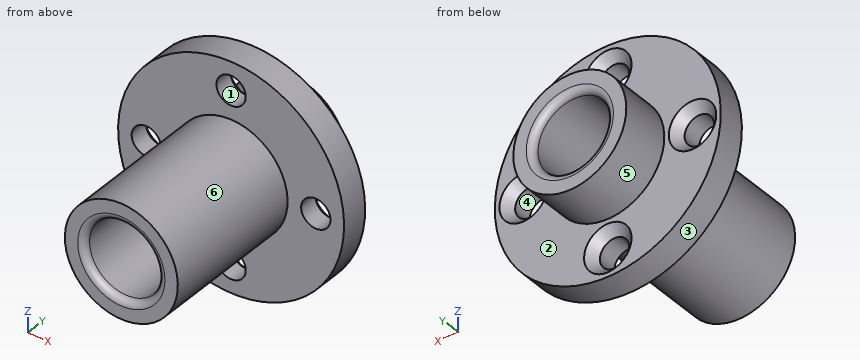
```python
from build123d import *

# Parameters (mm, degrees)
SKETCH2_R                    = 1.65
CUT_EXTRUDE1_DEPTH           = 27.647311778
CHAMFER1_SIZE                = 1.016
CIRPATTERN1_COUNT            = 4
CHAMFER1_OF_CIRPATTERN1_SIZE = 1.016
FILLET1_R                    = 0.762


with BuildPart() as part:
    # Sketch1 → Revolve1 (revolve)
    with BuildSketch(Plane.XY, mode=Mode.PRIVATE) as revolve1_sk:
        Polygon((4.1402, 12.7), (4.1402, -12.7), (6.35, -12.7), (6.35, 3.81), (12.7, 3.81), (12.7, 6.985), (6.35, 6.985), (6.35, 12.7), align=None)
    revolve(revolve1_sk.sketch.rotate(Axis((0, 0, 0), (0, -1, 0)), 90), axis=Axis((0, 0, 0), (0, -1, 0)))

    # Sketch2 → Cut-Extrude1 (cut, through all)
    with BuildSketch(Plane(origin=(0, 6.985, 0), x_dir=(1, 0, 0), z_dir=(0, 1, 0))):
        with Locations(Location((0, 9.525, 0), (0, 0, 270))):
            Circle(SKETCH2_R)
    cut_extrude1 = extrude(amount=-CUT_EXTRUDE1_DEPTH, mode=Mode.SUBTRACT)

    # Chamfer1
    chamfer1_edges = [part.edges().sort_by_distance(p)[0] for p in [
        (0, 6.985, -11.175),
    ]]
    chamfer(chamfer1_edges, length=CHAMFER1_SIZE)

    # CirPattern1: Cut-Extrude1 ×4 about axis
    cirpattern1_axis = Axis((0, 0, 0), (0, 1, 0))
    for i in range(1, CIRPATTERN1_COUNT):
        add(cut_extrude1.rotate(cirpattern1_axis, i * 360 / CIRPATTERN1_COUNT), mode=Mode.SUBTRACT)

    # Chamfer1 of CirPattern1
    chamfer1_of_cirpattern1_edges = [part.edges().sort_by_distance(p)[0] for p in [
        (-11.175, 6.985, 0),
        (0, 6.985, 11.175),
        (11.175, 6.985, 0),
    ]]
    chamfer(chamfer1_of_cirpattern1_edges, length=CHAMFER1_OF_CIRPATTERN1_SIZE)

    # Fillet1
    fillet1_edges = [part.edges().sort_by_distance(p)[0] for p in [
        (0, 12.7, -4.1402),
        (0, -12.7, -4.1402),
    ]]
    fillet(fillet1_edges, radius=FILLET1_R)


solid = part.part
```
Model file for the job. Use its own axes, mm. Face numbers are marked on the shaded views. A direction names the side the tool comes from. Round coordinates to 2 decimals unless told otherwise and drop trailing zeros. Write each loop counter-clockwise with the first axis right and the second up, starting at its lowest first coordinate (ties: lowest second). Pieces come first, ordered by that corner, then holes. Notation, with made-up numbers: M -13,-37 L 34,-37 A36 ccw 34,2 Z; hole C 21.5,79.25 d6. An arc over 180 degrees is marked long. Put each result on its own line as item: value.
Item 1: Probe L1, parallel to X at y = 3.75, z = 0; L2, parallel to Y at x = -6.5, z = -9.25 (3 decimals); L3, parallel to Z at x = -1.25, y = 2. List the from-to ranges inside material, lowest first. Write a range as from..to.
Responses:
L1: -6.35..-4.14, 4.14..6.35
L2: 3.81..6.985
L3: -6.23..-3.95, 3.95..6.23
Item 2: Cut at D-D (y = 2.5). List the corners of the cut face in (x, z), and give its area (3 significant figures).
Responses:
outline: C 0,0 d12.7; hole C 0,0 d8.28
area: 72.8 mm²
Item 3: Tool access for the marked faces 4, 5 and 6: list every direction of +Z, -Z, +X, -X, +Y, -Y with a clear straight run to the whole face (end or side of a thin tool).
Responses:
face 4: +Y, -Y
face 5: +Y
face 6: -Y
Item 4: Cut at C-C (x = 5.5). List the corners of the cut face in (y, z) (3 decimals), and give its area (3 significant figures).
Responses:
outline: M -12.7,-3.174 L 3.81,-3.174 L 3.81,-11.447 L 6.985,-11.447 L 6.985,-3.174 L 12.7,-3.174 L 12.7,3.174 L 6.985,3.174 L 6.985,11.447 L 3.81,11.447 L 3.81,3.174 L -12.7,3.174 Z
area: 214 mm²
Item 5: Cut at A-A (z = 0). State how many separate pieces and enclosed holes the cut face has, and give its area (3 significant figures).
Responses:
separate pieces: 4
enclosed holes: 0
area: 129 mm²
Item 6: Flat gauge pins, fed straight in: P1, Ø5, axis at y = 2, z = 5, coming from the -X side; P2, Ø3, axis at x = 0, z = 9.525, coming from the -Y side; P3, Ø4, axis at y = -3.5, z = 6, coming from the +X side; P4, Ø12.5, axis at x = 2.5, z = 6, coming from the -Y side. Where does each tip first touch, or does it go through?
Responses:
P1: x = -12.27
P2: through
P3: x = 4.93
P4: y = -12.7
Item 7: Mould opens along Z. For the marked faces 1, 2 and 3 say: +Z half, -Z half, draft (parallel to the pull), parting line (faces both ways), or undercut.
Responses:
face 1: undercut
face 2: draft
face 3: parting line
